```python
from build123d import *

# Parameters (mm, degrees)
CUT_EXTRUDE_1_DEPTH = 2
FILLET_1_R          = 0.3
CHAMFER_1_SIZE      = 0.3


with BuildPart() as part:
    # Эскиз1 → Повернуть1 (revolve)
    with BuildSketch(Plane(origin=(0, 0, 0), x_dir=(0, 0, -1), z_dir=(1, 0, 0))):
        Polygon((0, 0), (0, 2.3), (2, 2.3), (2, 1.5), (10, 1.5), (10, 0), align=None)
    revolve(axis=Axis((0, 0, 0), (0, 0, 1)))

    # Эскиз2 → Вырез-Вытянуть1 (cut)
    with BuildSketch(Plane.XY):
        Polygon((1.443375673, 0), (0.721687836, 1.25), (-0.721687836, 1.25), (-1.443375673, 0), (-0.721687836, -1.25), (0.721687836, -1.25), align=None)
    extrude(amount=-CUT_EXTRUDE_1_DEPTH, mode=Mode.SUBTRACT)

    # Скругление1
    fillet_1_edges = [part.edges().sort_by_distance(p)[0] for p in [
        (0, -1.5, -2),
    ]]
    fillet(fillet_1_edges, radius=FILLET_1_R)

    # Фаска1
    chamfer_1_edges = [part.edges().sort_by_distance(p)[0] for p in [
        (0, -1.5, -10),
    ]]
    chamfer(chamfer_1_edges, length=CHAMFER_1_SIZE)


solid = part.part
```
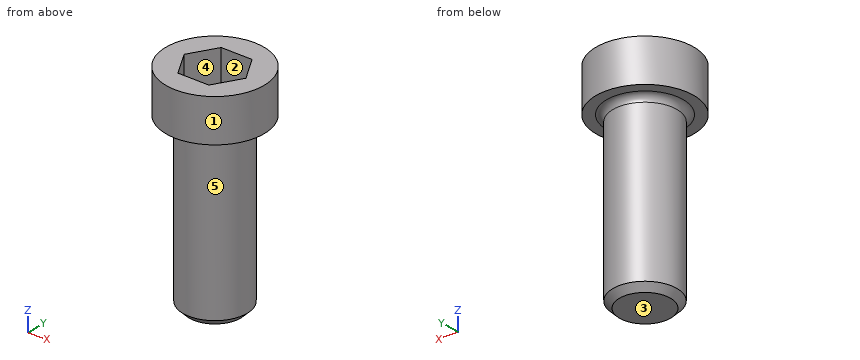
Read the model definition and answer for the solid it produces. Units are mm, in the model's axes. Face numbers are marked on the shaded views. A direction names the side the tool comes from. Coordinates: 2 decimals unless noted, no trailing zeros. Order: outer loops, then holes, each group sorted by start corner. A loop starts at its lowest first (then second) coordinate and runs counter-clockwise, first axis right, second up. Notation, with made-up numbers: (48.5, 45) - (95.5, 45) arc R20 ccw to (95.5, 79) - close; hole circle Ø2 at (12.25, 2.25). An arc over 180 degrees is marked (long way). Answer as a JSON object with one key per item and string values. Group by question number.
Item 1: Flat-ended cylindrical pins translate along their axes: P1, Ø1.5, axis at x = 0.5, z = -9, coming from the +Y side; P2, Ø1.5, axis at y = 1.5, z = -6, coming from the -X side; P3, Ø1.2, axis at x = 0.5, y = 0, coming from the +Z side. Find the tip coordinate at first contact, or state that the pin passes through.
Item 2: Section A-A (x = 0) is taken. Give the vertices of the cut face in (y, z).
Item 3: The mould has two halves that part along Y. Classify the marked faces 3, 4 and 5: +Y half, -Y half, draft (parallel to the pull), parting line (faces both ways), or undercut.
Item 4: Consider probe 1 along Z at (x, y) = (0.4, 0.1); probe 2 along Z at (x, y) = (0.2, -1.9); probe 3 along Y at (x, z) = (0.4, -9.5). Determine where each line is inside the solid, lowest interval first. Write a range as from..to.
Item 5: A tool of negligible diameter and unlimited length cuts with its end or side. For the marked faces 1 and 2, from which of +Z, -Z, +X, -X, +Y, -Y can it reach the whole face along a straight path? Write none if from no direction.
Results are:
{
 "1": {"P1": "stops at y = 1.5", "P2": "stops at x = -1.3", "P3": "stops at z = -2"},
 "2": {"outline": "(-2.3, -2) - (-1.8, -2) arc R0.3 cw to (-1.5, -2.3) - (-1.5, -9.7) - (-1.2, -10) - (1.2, -10) - (1.5, -9.7) - (1.5, -2.3) arc R0.3 cw to (1.8, -2) - (2.3, -2) - (2.3, 0) - (1.25, 0) - (1.25, -2) - (-1.25, -2) - (-1.25, 0) - (-2.3, 0) - close"},
 "3": {"face 3": "draft", "face 4": "undercut", "face 5": "parting line"},
 "4": {"probe 1": "z = -10..-2", "probe 2": "z = -2..0", "probe 3": "y = -1.45..1.45"},
 "5": {"face 1": "+Z, -Z", "face 2": "+Z"}
}
